Geometry check sheet. Reference: the model listing, model coordinates, mm. A direction names the side the tool comes from. Give positions to 0.01 mm unless a question says otherwise; leave off trailing zeros. Loops run counter-clockwise (first coordinate to the right, second up) from the corner with the lowest first, then second, coordinate; pieces in that order, holes last. Notation, with made-up numbers: (11, -4) -> (27, -4) arc R37 ccw to (27, 34) -> close; hole circle Ø8 at (-31.75, 28.5). An arc over 180 degrees is marked (long way). Write item = value, one per line. Start each with the question number.
Autodesk Inventor part; units mm, degrees
ref_plane "YZ Plane" through (0, 0, 0) normal (1, 0, 0) x (0, 1, 0)
ref_plane "XZ Plane" through (0, 0, 0) normal (0, 1, 0) x (-1, 0, 0)
ref_plane "XY Plane" through (0, 0, 0) normal (0, 0, 1) x (1, 0, 0)
sketch "Sketch1" plane through (0, 0, 0) normal (0, 1, 0) x (-1, 0, 0)
  circle A0 centre (0, 0) radius 4
  dimension "d0" = 8
extrude "Extrusion1" add sketch "Sketch1" along normal blind 10
sketch "Sketch2" plane through (0, 10, 0) normal (0, 1, 0) x (1, 0, 0)
  circle A0 centre (0, 0) radius 6.5
  dimension "d3" = 13
extrude "Extrusion2" add sketch "Sketch2" along normal blind 23
sketch "Sketch3" plane through (0, 33, 0) normal (0, 1, 0) x (1, 0, 0)
  circle A0 centre (0, 0) radius 4.5
  dimension "d6" = 9
hole "Hole1" at (0, 33, 0) direction (0, -1, 0) diameter 5 depth 40 tip angle 118 counterbore diameter 9 counterbore depth 18
properties part number "Exhaust Pipe Connector"
1) Tool access check on faces 4 (the flat face through (3, 10, -3)), 5 (the cylindrical face through (-4.46, 23.87, -0.59)), 6 (the flat face through (-2, 0, 2)). Record the directions out of +Z, -Z, +X, -X, +Y, -Y that give a thin tool (end or side, any length) a straight path to the whole face; none if there is none.
2) Depth check by flat-ended pin: pin 1 Ø5 at (y, z) = (22.5, -4.5) entering from -X; pin 2 Ø6 at (x, y) = (4.5, 18.5) entering from +Z; pin 3 Ø2 at (y, z) = (16, 3) entering from +X. Enter the tip coordinate at first touch or a pass-through.
3) Section check D-D (x = -3). Enter the section's corners in (y, z).
4) Thickness scan on line 1 (Z direction, x = 0, y = 5); line 2 (Z direction, x = 0, y = 19.25). Record the ranges inside material, lowest first.
5) Section check C-C (y = 4). Enter the section's corners in (x, z), plus the area to 3 significant figures.
6) Section check B-B (z = 0). Enter the section's corners in (x, y).
7) Draft check along Z on faces 1 (the flat face through (-1.54, 33, -4.42)), 2 (the cylindrical face through (2.44, 7.4, -0.54)), 3 (the cylindrical face through (-5.158, 21.339, -3.955)). Enter one of: released by +Z, released by -Z, zero draft, split by the parting line, or undercut.
8) Section check A-A (x = 0). Enter the section's corners in (y, z), plus the area to 3 significant figures.
Check result:
q1.face_4 = -Y
q1.face_5 = +Y
q1.face_6 = +Z, -Z, +X, -X, -Y
q2.pin_1 = -6.18
q2.pin_2 = 6.32
q2.pin_3 = 6.18
q3.outline = (0, -2.65) -> (10, -2.65) -> (10, -5.77) -> (33, -5.77) -> (33, -3.35) -> (15, -3.35) -> (15, 3.35) -> (33, 3.35) -> (33, 5.77) -> (10, 5.77) -> (10, 2.65) -> (0, 2.65) -> close
q4.line_1 = -4 to -2.5, 2.5 to 4
q4.line_2 = -6.5 to -4.5, 4.5 to 6.5
q5.outline = circle Ø8 at (0, 0); hole circle Ø5 at (0, 0)
q5.area = 30.6 mm2
q6.outline = (-6.5, 10) -> (-4, 10) -> (-4, 0) -> (-2.5, 0) -> (-2.5, 15) -> (-4.5, 15) -> (-4.5, 33) -> (-6.5, 33) -> close; (2.5, 0) -> (4, 0) -> (4, 10) -> (6.5, 10) -> (6.5, 33) -> (4.5, 33) -> (4.5, 15) -> (2.5, 15) -> close
q7.face_1 = zero draft
q7.face_2 = undercut
q7.face_3 = split by the parting line
q8.outline = (0, -4) -> (10, -4) -> (10, -6.5) -> (33, -6.5) -> (33, -4.5) -> (15, -4.5) -> (15, -2.5) -> (0, -2.5) -> close; (0, 2.5) -> (15, 2.5) -> (15, 4.5) -> (33, 4.5) -> (33, 6.5) -> (10, 6.5) -> (10, 4) -> (0, 4) -> close
q8.area = 142 mm2
